The model under review builds one solid part; all positions refer to its coordinate system, in mm. Face numbers are marked on the shaded views. Coordinates: 2 decimals unless noted, no trailing zeros. Order: outer loops, then holes, each group sorted by start corner. A loop starts at its lowest first (then second) coordinate and runs counter-clockwise, first axis right, second up. Notation, with made-up numbers: (-23, 89.5) - (-18, 89.5) arc R19 ccw to (-18, 121.5) - close; hole circle Ø5 at (39, 49). An arc over 180 degrees is marked (long way). Answer in a Markdown table with one row per item.
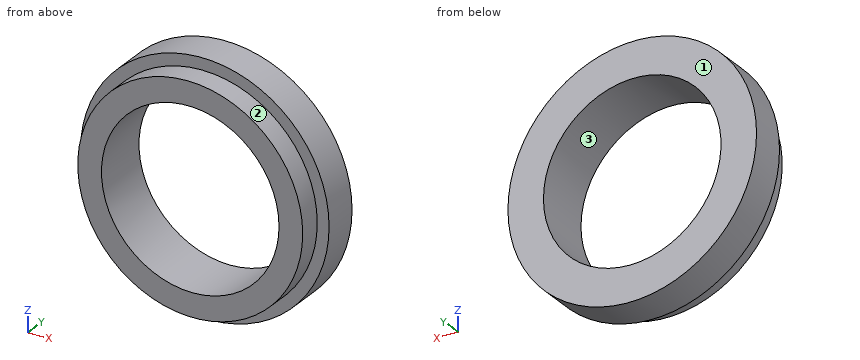
```python
from build123d import *

# Parameters (mm, degrees)
SCHIZZO1_R                   = 9.5
SCHIZZO1_R_2                 = 7.5
ESTRUSIONE_ESTRUSIONE1_DEPTH = 5
SCHIZZO2_R                   = 10.5
SCHIZZO2_R_2                 = 9.5
ESTRUSIONE_ESTRUSIONE2_DEPTH = 3
SCHIZZO3_R                   = 9.5
TAGLIO_ESTRUSIONE1_DEPTH     = 0.1


with BuildPart() as part:
    # Schizzo1 → Estrusione-Estrusione1 (new body)
    with BuildSketch(Plane(origin=(0, 0, 0), x_dir=(1, 0, 0), z_dir=(0, 1, 0))):
        Circle(SCHIZZO1_R)
        Circle(SCHIZZO1_R_2, mode=Mode.SUBTRACT)
    extrude(amount=ESTRUSIONE_ESTRUSIONE1_DEPTH)

    # Schizzo2 → Estrusione-Estrusione2 (add)
    with BuildSketch(Plane(origin=(0, 5, 0), x_dir=(1, 0, 0), z_dir=(0, 1, 0))):
        Circle(SCHIZZO2_R)
        Circle(SCHIZZO2_R_2, mode=Mode.SUBTRACT)
    extrude(amount=-ESTRUSIONE_ESTRUSIONE2_DEPTH)

    # Schizzo3 → Taglio-Estrusione1 (cut)
    with BuildSketch(Plane.XZ):
        Circle(SCHIZZO3_R)
    extrude(amount=-TAGLIO_ESTRUSIONE1_DEPTH, mode=Mode.SUBTRACT)


solid = part.part
```
Item 1: To check wall thickness, follow line 1 (Z direction, x = 0, y = 1.85); line 2 (Z direction, x = 0, y = 3.8). State the ranges of each line that lie inside material, in increasing order. Write a range as from..to.
Check values:
| item | result |
|---|---|
| line 1 | -9.5..-7.5, 7.5..9.5 |
| line 2 | -10.5..-7.5, 7.5..10.5 |
Item 2: We need section A-A, the plane x = 0. Write out the cut boundary in (y, z).
Check values:
| item | result |
|---|---|
| outline | (0.1, -9.5) - (2, -9.5) - (2, -10.5) - (5, -10.5) - (5, -7.5) - (0.1, -7.5) - close; (0.1, 7.5) - (5, 7.5) - (5, 10.5) - (2, 10.5) - (2, 9.5) - (0.1, 9.5) - close |
Item 3: Clearance check with a flat-ended pin moving along its axis: pin 1 Ø1 at (x, y) = (4, 2) entering from -Z. State where the tip first meets the part, or that it passes through.
Check values:
| item | result |
|---|---|
| pin 1 | z = -9.9 |
Item 4: We need section D-D, the plane y = 0.8. Write out the cut boundary in (x, z).
Check values:
| item | result |
|---|---|
| outline | circle Ø19 at (0, 0); hole circle Ø15 at (0, 0) |
Item 5: We need section C-C, the plane x = 8.25. Write out the cut boundary in (y, z).
Check values:
| item | result |
|---|---|
| outline | (0.1, -4.71) - (2, -4.71) - (2, -6.5) - (5, -6.5) - (5, 6.5) - (2, 6.5) - (2, 4.71) - (0.1, 4.71) - close |
Item 6: Mouldability with a two-part tool opening along X and no side actions: class the marked faces 1, 2 and 3 as +X half, -X half, draft (parallel to the pull), parting line (faces both ways), or undercut.
Check values:
| item | result |
|---|---|
| face 1 | draft |
| face 2 | parting line |
| face 3 | undercut |
Item 7: We need section B-B, the plane z = 0. Write out the cut boundary in (x, y).
Check values:
| item | result |
|---|---|
| outline | (-10.5, 2) - (-9.5, 2) - (-9.5, 0.1) - (-7.5, 0.1) - (-7.5, 5) - (-10.5, 5) - close; (7.5, 0.1) - (9.5, 0.1) - (9.5, 2) - (10.5, 2) - (10.5, 5) - (7.5, 5) - close |
